Here's the drawing with two shaded views (mm, measured from the low corner). I have some questions. A direction names the side the tool comes from. Coordinates: 2 decimals unless noted, no trailing zeros. Write each loop counter-clockwise with the first axis right and the second up, starting at its lowest first coordinate (ties: lowest second). Pieces come first, ordered by that corner, then holes.
Item 1: I want a section at D-D on x = 291.5. Please give me the cut outline in (y, z) (1 decimal).
Item 2: If I drill on probe 1 along Z at (x, y) = (9.5, 15); probe 2 along X at (y, z) = (24.5, 9.75); probe 3 along X at (y, z) = (167, 17.25), over which ranges is the centre line in solid material (lowest first)?
Item 3: I want a section at C-C on y = 186.5. Please give me the cut outline in (x, z).
Item 4: Thinking about a two-plate mould opening in X: for the marked faces 1, 2 and 3, which applies, +X half, -X half, draft (parallel to the pull), parting line (faces both ways), or undercut?
Item 5: For P1, Ø1, axis at y = 164, z = 10.5, coming from the +X side; P2, Ø8, axis at x = 154, z = 3.5, coming from the -Y side; P3, Ø7, axis at y = 15, z = 10, coming from the +X side; P4, Ø5, axis at y = 68, z = 8.5, coming from the +X side, each with a flat end and sliding along its axis, tell me the tip position at first contact or that it passes through.
Item 6: I want a section at A-A on y = 15. Please give me the cut outline in (x, z).
Item 7: Which directions (+Z, -Z, +X, -X, +Y, -Y) give clear straight access to the entire face, cutting with the end or side of a thin tool? Please do the marked faces 4 and 5.
Item 8: I want a section at B-B on y = 52. Please give me the cut outline in (x, z) (1 decimal).
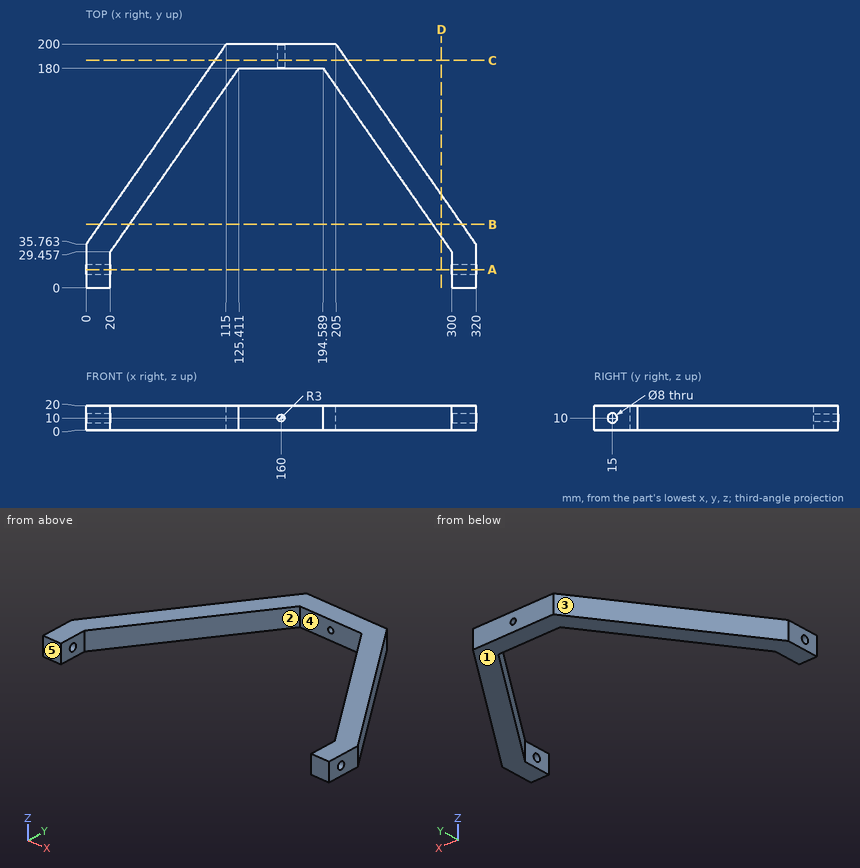
Response values:
1. outline: (41.6, 0) - (76.5, 0) - (76.5, 20) - (41.6, 20) - close
2. probe 1: z = 0 to 6, 14 to 20
2. probe 2: x = 0 to 20, 300 to 320
2. probe 3: x = 91.89 to 116.31, 203.69 to 228.11
3. outline: (105.55, 0) - (214.45, 0) - (214.45, 20) - (105.55, 20) - close; hole circle Ø6 at (160, 10)
4. face 1: draft
4. face 2: undercut
4. face 3: -X half
5. P1: stops at x = 230.56
5. P2: stops at y = 180
5. P3: passes through
5. P4: stops at x = 299.18
6. outline: (0, 0) - (20, 0) - (20, 6) - (0, 6) - close; (0, 14) - (20, 14) - (20, 20) - (0, 20) - close; (300, 0) - (320, 0) - (320, 6) - (300, 6) - close; (300, 14) - (320, 14) - (320, 20) - (300, 20) - close
7. face 4: +Z, -Z, -Y
7. face 5: +Z, -Z, +X, -X, -Y
8. outline: (11.4, 0) - (35.8, 0) - (35.8, 20) - (11.4, 20) - close; (284.2, 0) - (308.6, 0) - (308.6, 20) - (284.2, 20) - close
